Source: three-view drawing plus pictorial views. Frame: mm from the lowest corner of the part. Round coordinates to 2 decimals unless told otherwise and drop trailing zeros. Loops run counter-clockwise (first coordinate to the right, second up) from the corner with the lowest first, then second, coordinate; pieces in that order, holes last. Notation, with made-up numbers: (-16, 64.5) -> (-2, 64.5) arc R26 cw to (-2, 98.5) -> close; hole circle Ø4 at (-29, 71). An arc over 180 degrees is marked (long way). Answer in a Markdown table with one row per item. Add a question column.
Q1. Section C-C, the plane z = 14. Output: boundary loops of the cut face in (x, y).
Q2. Section A-A, the plane x = 202. Output: boundary loops of the cut face in (y, z).
Q3. Pin query (flat end, axial travel): pin 1 (4 mm diameter, centred on x = 227.5, y = 8, fed in from -Z); pin 2 (6 mm diameter, centred on y = 3, z = 58.5, fed in from -X); pin 3 (5 mm diameter, centred on y = 6.5, z = 21.5, fed in from -X); pin 4 (5 mm diameter, centred on x = 189.5, y = 6.5, fed in from +Z). Return the tip coordinate at first contact, or that it passes through.
Q4. Ray query, L1, parallel to Z at x = 134.5, y = 4; L2, parallel to X at y = 6.75, z = 85.5; L3, parallel to X at y = 3, z = 6. Return the intervals inside material, ascending. Write a range as from..to.
Q5. Section B-B, the plane y = 7.5. Output: boundary loops of the cut face in (x, z), and give its area (3 significant figures).
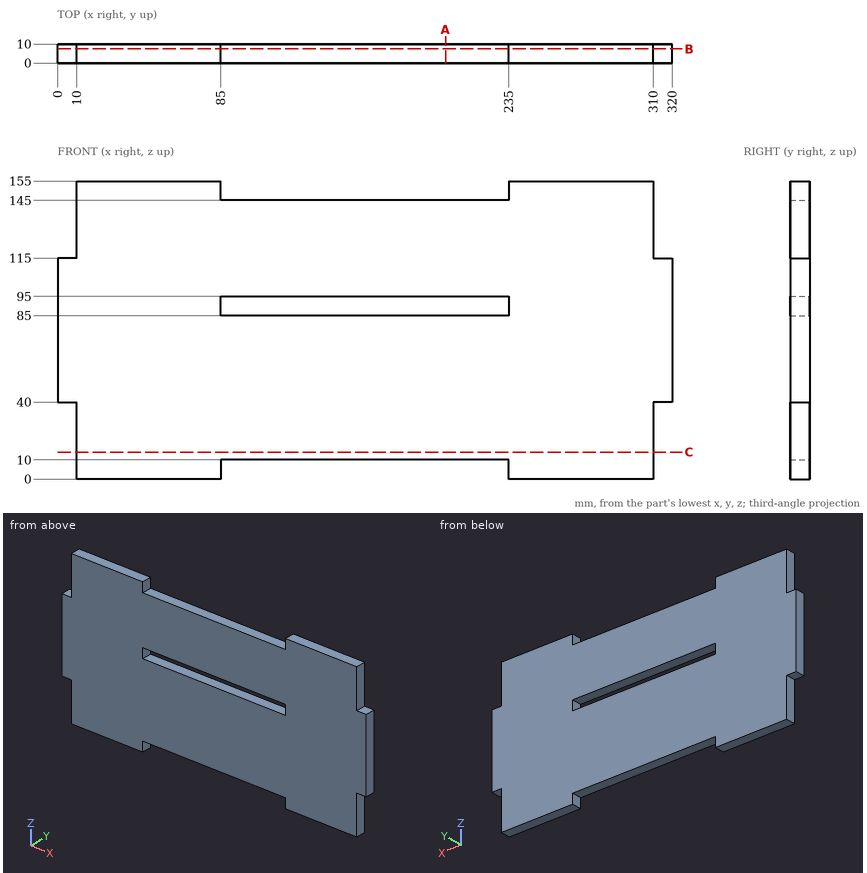
Answer block:
| question | item | result |
|---|---|---|
| 1 | outline | (10, 0) -> (310, 0) -> (310, 10) -> (10, 10) -> close |
| 2 | outline | (0, 10) -> (10, 10) -> (10, 85) -> (0, 85) -> close; (0, 95) -> (10, 95) -> (10, 145) -> (0, 145) -> close |
| 3 | pin 1 | z = 10 |
| 3 | pin 2 | x = 0 |
| 3 | pin 3 | x = 10 |
| 3 | pin 4 | z = 145 |
| 4 | L1 | 10..85, 95..145 |
| 4 | L2 | 0..85, 235..320 |
| 4 | L3 | 10..85, 235..310 |
| 5 | outline | (0, 40) -> (10, 40) -> (10, 0) -> (85, 0) -> (85, 10) -> (235, 10) -> (235, 0) -> (310, 0) -> (310, 40) -> (320, 40) -> (320, 115) -> (310, 115) -> (310, 155) -> (235, 155) -> (235, 145) -> (85, 145) -> (85, 155) -> (10, 155) -> (10, 115) -> (0, 115) -> close; hole (85, 85) -> (235, 85) -> (235, 95) -> (85, 95) -> close |
| 5 | area | 43,500 mm^2 |
